The listing builds one solid part. Answer for the finished solid, in the listing's coordinates (mm). Face numbers are marked on the shaded views. Coordinates: 2 decimals unless noted, no trailing zeros. Write each loop counter-clockwise with the first axis right and the second up, starting at its lowest first coordinate (ties: lowest second). Pieces come first, ordered by that corner, then holes.
(1) The part is cut by section C-C on z = 5. Determine the outline of the cut face in (x, y).
(2) The part is cut by section D-D on y = 2.75. Determine the outline of the cut face in (x, z), plus the area to 3 significant figures.
(3) The part is cut by section B-B on y = 0. Determine the outline of the cut face in (x, z), plus the area to 3 significant figures.
(4) Given P1, Ø3, axis at x = 0, z = -5, coming from the +Y side, flat-ended and moving along its own axis, determine where the tip first touches the part or whether it passes through.
(5) The part is cut by section A-A on x = 0. Determine the outline of the cut face in (y, z), plus the area to 3 significant figures.
(6) Straight lines are drawn through the part: line 1 (X direction, y = -0.5, z = -5); line 2 (Z direction, x = 2, y = 0.5). For each, find the intervals that lie inside material, in ascending order.
(7) For a pull along Z with two mould halves and no side action, classify the marked faces 1, 2 and 3 as +Z half, -Z half, draft (parallel to the pull), parting line (faces both ways), or undercut.
from build123d import *

# Parameters (mm, degrees)
SKETCH_1_W      = 8
SKETCH_1_H      = 8
EXTRUDE_1_DEPTH = 20
HOLE_WIZARD_1_D = 2.5
HOLE_WIZARD_2_D = 2.5
CHAMFER_1_SIZE  = 0.3


with BuildPart() as part:
    # 草图1 → 凸台-拉伸1 (new, symmetric)
    with BuildSketch(Plane.XY):
        Rectangle(SKETCH_1_W, SKETCH_1_H)
    extrude(amount=EXTRUDE_1_DEPTH, both=True)

    # Hole Wizard 1 (through all)
    with Locations(Plane.ZY.offset(4)):
        with Locations((-15, 0), (5, 0)):
            Hole(HOLE_WIZARD_1_D / 2)

    # Hole Wizard 2 (through all)
    with Locations(Plane(origin=(0, 4, 0), x_dir=(1, 0, 0), z_dir=(0, 1, 0))):
        with Locations((0, 5), (0, -15)):
            Hole(HOLE_WIZARD_2_D / 2)

    # 倒角1
    chamfer_1_edges = [part.edges().sort_by_distance(p)[0] for p in [
        (-4, 0, 20),
        (0, -4, 20),
        (4, 0, 20),
        (0, -4, -20),
        (-4, 0, -20),
        (4, 0, -20),
        (4, -4, 0),
        (-4, -4, 0),
        (-4, 4, 0),
        (4, 4, 0),
        (0, 4, 20),
    ]]
    chamfer(chamfer_1_edges, length=CHAMFER_1_SIZE)


solid = part.part
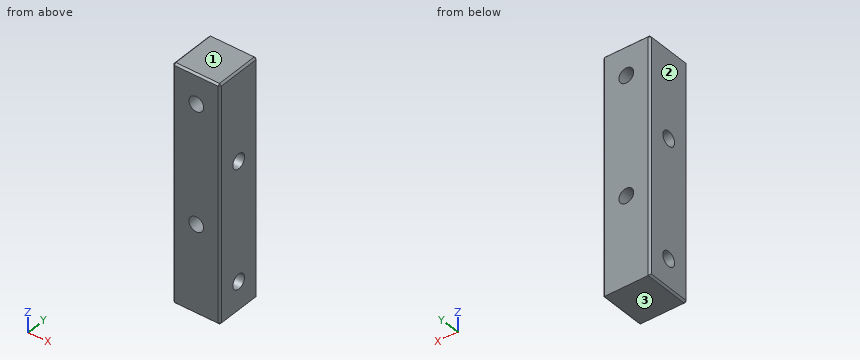
Model answer:
1. outline: (-4, -3.7) - (-3.7, -4) - (3.7, -4) - (4, -3.7) - (4, -1.25) - (-4, -1.25) - close; (-4, 1.25) - (4, 1.25) - (4, 3.7) - (3.7, 4) - (-3.7, 4) - (-4, 3.7) - close
2. outline: (-4, -19.7) - (-3.7, -20) - (3.7, -20) - (4, -19.7) - (4, 19.7) - (3.7, 20) - (-3.7, 20) - (-4, 19.7) - close; hole circle Ø2.5 at (0, -5); hole circle Ø2.5 at (0, 15)
2. area: 310 mm2
3. outline: (-4, -19.7) - (-3.7, -20) - (3.7, -20) - (4, -19.7) - (4, -16.25) - (-4, -16.25) - close; (-4, -13.75) - (4, -13.75) - (4, 3.75) - (-4, 3.75) - close; (-4, 6.25) - (4, 6.25) - (4, 19.7) - (3.7, 20) - (-3.7, 20) - (-4, 19.7) - close; hole circle Ø2.5 at (0, -5); hole circle Ø2.5 at (0, 15)
3. area: 270 mm2
4. P1: stops at y = 4
5. outline: (-4, -19.7) - (-3.7, -20) - (4, -20) - (4, -6.25) - (-4, -6.25) - close; (-4, -3.75) - (4, -3.75) - (4, 13.75) - (-4, 13.75) - close; (-4, 16.25) - (4, 16.25) - (4, 19.7) - (3.7, 20) - (-3.7, 20) - (-4, 19.7) - close; hole circle Ø2.5 at (0, -15); hole circle Ø2.5 at (0, 5)
5. area: 270 mm2
6. line 1: x = -4 to -1.25, 1.25 to 4
6. line 2: z = -20 to -16.15, -13.85 to 3.85, 6.15 to 20
7. face 1: +Z half
7. face 2: draft
7. face 3: -Z half
